Autodesk Inventor part; units mm, degrees
ref_plane "YZ Plane" through (0, 0, 0) normal (1, 0, 0) x (0, 1, 0)
ref_plane "XZ Plane" through (0, 0, 0) normal (0, 1, 0) x (-1, 0, 0)
ref_plane "XY Plane" through (0, 0, 0) normal (0, 0, 1) x (1, 0, 0)
sketch "Sketch1" plane through (0, 0, 0) normal (0, 1, 0) x (-1, 0, 0)
  line L0 (0, 0) -> (40.005, 0)
  line L1 (40.005, 0) -> (40.005, -40.0202)
  line L2 (40.005, -40.0202) -> (0, -40.0202)
  line L3 (0, -40.0202) -> (0, 0)
  dimension "d26" = 40.005
  dimension "d27" = 40.0202
extrude "Extrusion1" add sketch "Sketch1" along normal blind 4
sketch "Sketch2" plane through (0, 4, 0) normal (0, 1, 0) x (1, 0, 0)
  line L0 (-40.0202, 0) -> (0, 0)
  line L1 (0, 0) -> (0, 40)
  line L2 (0, 40) -> (-40.0202, 40)
  line L3 (-40.0202, 40) -> (-40.0202, 0)
  line L4 (-37.0202, 37) -> (-3, 37)
  line L5 (-3, 37) -> (-3, 3)
  line L6 (-3, 3) -> (-37.0202, 3)
  line L7 (-37.0202, 3) -> (-37.0202, 37)
  circle A0 centre (-37.0202, 37) radius 1.5
  circle A1 centre (-3, 37) radius 1.5
  circle A2 centre (-3, 3) radius 1.5
  circle A3 centre (-37.0202, 3) radius 1.5
  dimension "d4" = 3
  dimension "d5" = 3
  dimension "d6" = 3
  dimension "d7" = 3
  dimension "d8" = 3
extrude "Extrusion2" cut sketch "Sketch2" against normal blind 4 contours L7 A0 L4 | L4 A0 L7 | A1 L5 L4 | L4 L5 A1 | A3 L6 L7 | L7 L6 A3 | A2 L6 L5 | L5 L6 A2
sketch "Sketch3" plane through (0, 4, 0) normal (0, 1, 0) x (1, 0, 0)
  circle A0 centre (-37.0202, 3) radius 1.5
  circle A1 centre (-37.0202, 37) radius 1.5
  circle A2 centre (-3, 37) radius 1.5
  circle A3 centre (-3, 3) radius 1.5
  circle A4 centre (-37.0202, 3) radius 1.5
  circle A5 centre (-3, 37) radius 1.5
  circle A6 centre (-37.0202, 37) radius 1.5
  circle A7 centre (-3, 3) radius 1.5
  line L0 (-40.005, 0) -> (0, 0)
  line L1 (0, 0) -> (0, 40.0202)
  line L2 (0, 40.0202) -> (-40.005, 40.0202)
  line L3 (-40.005, 40.0202) -> (-40.005, 0)
  circle A8 centre (-3, 37) radius 3
  circle A9 centre (-3, 3) radius 3
  circle A10 centre (-37.0202, 3) radius 3
  circle A11 centre (-37.0202, 37) radius 2.9848
extrude "Extrusion3" add sketch "Sketch3" along normal blind 1.5 contours A8 | A11 | A10 L3 | A10 L3 | A9
sketch "Sketch4" plane through (0, 0, 0) normal (0, -1, 0) x (1, 0, 0)
  circle A0 centre (-3, -37) radius 1.5
  circle A1 centre (-37.0202, -37) radius 1.5
  circle A2 centre (-37.0202, -3) radius 1.5
  circle A3 centre (-3, -3) radius 1.5
  circle A4 centre (-3, -3) radius 2.5
  circle A5 centre (-3, -37) radius 2.5
  circle A6 centre (-37.0202, -37) radius 2.5
  circle A7 centre (-37.0202, -3) radius 2.5
  point P0 (0, 0)
  dimension "d14" = 5
  dimension "d15" = 5
  dimension "d16" = 5
  dimension "d17" = 5
extrude "Extrusion4" cut sketch "Sketch4" against normal blind 3
fillet "Fillet2" radius 3 4 edges at (-40.005, 2, -40.0202) (-40.005, 2, 0) (0, 2, 0) (0, 2, -40.0202)
sketch "Sketch7" plane through (0, 0, -3) normal (1, 0, 0) x (0, 0, -1)
  line L0 (34.0202, 4) -> (34.0202, 0)
  line L1 (0, 0) -> (34.0202, 0)
  line L2 (34.0202, 0) -> (34.0202, 2)
  line L3 (34.0202, 2) -> (0, 2)
  line L4 (0, 2) -> (0, 0)
  point P0 (-3, 0)
  dimension "d29" = 2
extrude "Extrusion7" add sketch "Sketch7" along normal blind 3
sketch "Sketch8" plane through (-40.005, 4, -37) normal (-1, 0, 0) x (0, 0, 1)
  line L0 (34, -4) -> (-0.0202, -4)
  line L1 (-0.0202, -4) -> (-0.0202, -2)
  line L2 (-0.0202, -2) -> (34, -2)
  line L3 (34, -2) -> (34, -4)
  point P0 (37, -4)
extrude "Extrusion8" add sketch "Sketch8" along normal blind 3
properties part number "L298N-holder"
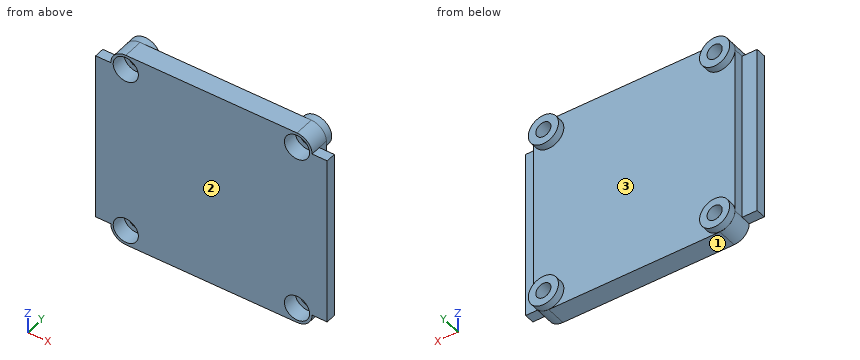
Geometry check sheet. Reference: the model listing, model coordinates, mm. Face numbers are marked on the shaded views. Coordinates: 2 decimals unless noted, no trailing zeros. Order: outer loops, then holes, each group sorted by start corner. A loop starts at its lowest first (then second) coordinate and runs counter-clockwise, first axis right, second up. Notation, with made-up numbers: (52, 62) - (107, 62) arc R18 cw to (107, 89) - close; hole circle Ø5 at (54.25, -4). An arc over 180 degrees is marked (long way). Answer in a Markdown table with one row per item. Add a question column.
1) Cross-section at A-A, the plane z = -8.5. Record the cut outline in (x, y) (3 decimals).
2) Cross-section at B-B, the plane x = -27.5. Record the cut outline in (y, z), then the cut area to 3 significant figures.
3) Release check for a two-part mould opening along Z. For the marked faces 1, 2 and 3 record: +Z half, -Z half, draft (parallel to the pull), parting line (faces both ways), or undercut.
4) Material ranges on line 1 along Z through (x, y) = (-3, 3.75); line 2 along X through (y, z) = (4.9, -37) (3 decimals); line 3 along X through (y, z) = (3.6, -3) (3 decimals), recorded low to high. Write a range as [from, to].
5) Gauge pin test, flat ends, axial feed: P1, Ø1.5, axis at x = -38, z = -37, coming from the -Y side; P2, Ø12, axis at x = -22.5, z = -27, coming from the +Y side; P3, Ø2, axis at y = 3.5, z = -24.5, coming from the +X side. Record the tip position at first contact, or that the pin passes through.
Check result:
| question | item | result |
|---|---|---|
| 1 | outline | (-43.005, 0) - (3, 0) - (3, 2) - (0, 2) - (0, 4) - (-40.005, 4) - (-40.005, 2) - (-43.005, 2) - close |
| 2 | outline | (0, -40.02) - (4, -40.02) - (4, 0) - (0, 0) - close |
| 2 | area | 160 mm² |
| 3 | face 1 | -Z half |
| 3 | face 2 | draft |
| 3 | face 3 | undercut |
| 4 | line 1 | z = [-40.02, -38.5], [-35.5, -4.5], [-1.5, 0] |
| 4 | line 2 | x = [-40.005, -38.52], [-35.52, -34.035], [-6, -4.5], [-1.5, 0] |
| 4 | line 3 | x = [-40.005, -38.52], [-35.52, -4.5], [-1.5, 0] |
| 5 | P1 | stops at y = 3 |
| 5 | P2 | stops at y = 4 |
| 5 | P3 | stops at x = 0 |
